```python
from build123d import *

# Parameters (mm, degrees)
SKETCH_1_R        = 7.9375
SKETCH_1_R_2      = 3.975
EXTRUDE_1_DEPTH   = 550.8625
FILLET_1_R        = 2.5
MOVE_BODY_1_ANGLE = 90


with BuildPart() as part:
    # 스케치1 → 보스-돌출1 (new body, symmetric)
    with BuildSketch(Plane(origin=(0, 0, 0), x_dir=(1, 0, 0), z_dir=(0, 1, 0))):
        Circle(SKETCH_1_R)
        Circle(SKETCH_1_R_2, mode=Mode.SUBTRACT)
    extrude(amount=EXTRUDE_1_DEPTH, both=True)

    # 필렛1
    fillet_1_edges = [part.edges().sort_by_distance(p)[0] for p in [
        (-7.9375, -550.8625, 0),
        (-7.9375, 550.8625, 0),
    ]]
    fillet(fillet_1_edges, radius=FILLET_1_R)


with BuildPart() as part_1:
    # Move Body 1: moved
    add(part.part.rotate(Axis((0, 0, 0), (0, 0, 1)), MOVE_BODY_1_ANGLE))


solid = part_1.part
```
Model file for the job. Use its own axes, mm. Coordinates: 2 decimals unless noted, no trailing zeros. Order: outer loops, then holes, each group sorted by start corner. A loop starts at its lowest first (then second) coordinate and runs counter-clockwise, first axis right, second up. Notation, with made-up numbers: (71.25, -0.5) -> (128.25, -0.5) arc R25 cw to (128.25, 35.5) -> close; hole circle Ø11 at (-16.5, 65.5). An arc over 180 degrees is marked (long way). Answer as a JSON object with one key per item and string values. Group by question number.
1) Drill centre lines: L1, parallel to Y at x = 8, z = 1.25; L2, parallel to Z at x = -98, y = 0 (1 decimal). Where is each one in solid material? Low to high.
2) Cut at A-A, the plane z = 0. Write the cut outline in (x, y) (1 decimal), then the cut area to 3 significant figures.
3) Flat gauge pins, fed straight in: pin 1 (5 mm diameter, centred on x = 256, y = 5.5, fed in from -Z); pin 2 (1 mm diameter, centred on x = -414.5, z = -5, fed in from -Y); pin 3 (1.5 mm diameter, centred on x = -237.5, z = 2.5, fed in from +Y); pin 4 (5 mm diameter, centred on x = -103, z = 2, fed in from -Y). Where does each tip first touch, or does it go through?
Check values:
{
 "1": {"L1": "y = -7.84 to -3.77, 3.77 to 7.84", "L2": "z = -7.9 to -4, 4 to 7.9"},
 "2": {"outline": "(-550.9, -5.4) arc R2.5 ccw to (-548.4, -7.9) -> (548.4, -7.9) arc R2.5 ccw to (550.9, -5.4) -> (550.9, -4) -> (-550.9, -4) -> close; (-550.9, 4) -> (550.9, 4) -> (550.9, 5.4) arc R2.5 ccw to (548.4, 7.9) -> (-548.4, 7.9) arc R2.5 ccw to (-550.9, 5.4) -> close", "area": "8,730 mm²"},
 "3": {"pin 1": "stops at z = -7.35", "pin 2": "stops at y = -6.54", "pin 3": "stops at y = 7.74", "pin 4": "stops at y = -7.94"}
}
